Source: CAD feature listing. Evaluate the final solid. Frame: model axes, mm. Give positions to 0.01 mm unless a question says otherwise; leave off trailing zeros. Write each loop counter-clockwise with the first axis right and the second up, starting at its lowest first coordinate (ties: lowest second). Pieces come first, ordered by that corner, then holes. Notation, with made-up numbers: M 43.25,68 L 58.25,68 A25 cw 58.25,92 Z; hole C -35,38 d4. An arc over 180 degrees is marked long. Return JSON: item names as keys, results as strings.
```python
from build123d import *

# Parameters (mm, degrees)
F0_W     = 55
F0_H     = 64
F1_DEPTH = 5
F2_SIZE  = 4.99999


# Not quite as in the source:
# - a fillet or chamfer is up to 0.001 mm smaller than in the source, because OpenCascade refuses the exact size


with BuildPart() as f1:
    # F0 (on Top) → F1 (new body)
    with BuildSketch(Plane.XY):
        with Locations((0, 20.5)):
            Rectangle(F0_W, F0_H)
    extrude(amount=F1_DEPTH)

    # F2 (size 5 in the source; OpenCascade refuses exactly that, so slightly less here)
    f2_edges = [f1.edges().sort_by_distance(p)[0] for p in [
        (-27.5, 20.5, 5),
        (0, 52.5, 5),
        (27.5, 20.5, 5),
    ]]
    chamfer(f2_edges, length=F2_SIZE)


solid = f1.part
```
1) Line query: line 1 (X direction, y = 38, z = 3.95); line 2 (Y direction, x = 4, z = 2.45); line 3 (Z direction, x = 23.5, y = 6). Output: solid intervals per line, ascending. Write a range as [from, to].
Numbers:
{"line 1": "x = [-23.55, 23.55]", "line 2": "y = [-11.5, 50.05]", "line 3": "z = [0, 4]"}
2) Contact query for flat-ended pins moving along their axis: pin 1 Ø3 at (y, z) = (0, 3.5) entering from -X; pin 2 Ø3 at (x, z) = (-9.5, 3) entering from +Y; pin 3 Ø1 at (x, y) = (-7.5, 2.5) entering from -Z. Output: stop coordinate, or through.
Numbers:
{"pin 1": "stops at x = -25.5", "pin 2": "stops at y = 51", "pin 3": "stops at z = 0"}
3) Cut plane C-C, the plane z = 2.4. Return the cut outline in (x, y), then the cut area to 3 significant figures.
Numbers:
{"outline": "M -25.1,-11.5 L 25.1,-11.5 L 25.1,50.1 L -25.1,50.1 Z", "area": "3,090 mm²"}
